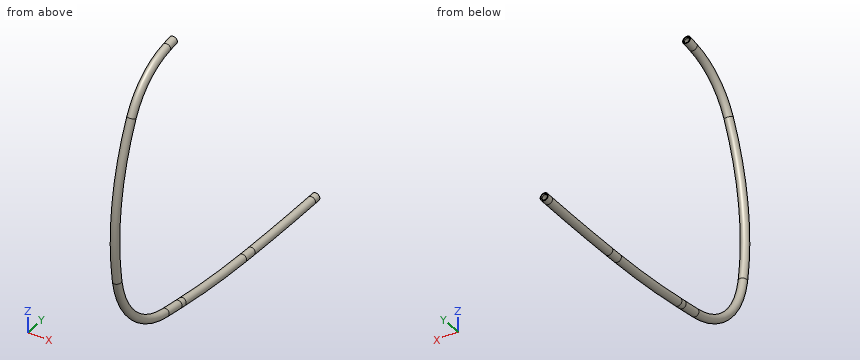
from build123d import *
from OCP.BRepFilletAPI import BRepFilletAPI_MakeChamfer

# Parameters (mm, degrees)
PERFIL_BOWDEN_R   = 3
PERFIL_BOWDEN_R_2 = 2
CHAFL_N2_SIZE     = 0.4
CHAFL_N2_SIZE2    = 0.692820323


with BuildPart() as part:
    # Barrer1: sweep along a curve in space
    with BuildLine() as barrer1_path:
        Line((-179.55, 237.9, 23.45), (-179.55, 232.9, 23.45))
        ThreePointArc((-179.55, 232.9, 23.45), (-179.55, 197.994333352, 23.830077258), (-179.55, 163.105218927, 24.970128802))
        ThreePointArc((-179.55, 163.105218927, 24.970128802), (-179.55, 158.110113707, 25.191344172), (-179.55, 153.115325109, 25.419596817))
        ThreePointArc((-179.55, 153.115325109, 25.419596817), (-179.55, 117.985550969, 28.025652191), (-179.55, 83.053766812, 32.571310699))
        Line((-179.55, 78.115325109, 33.353483024), (-179.55, 83.053766812, 32.571310699))
        Line((-179.55, 78.115325109, 33.353483024), (-179.55, 63.3, 35.7))
        ThreePointArc((-179.55, 63.3, 35.7), (-179.431411326, 26.758540491, 54.415674643), (-179.12153359, 8.351916444, 91.11266322))
        ThreePointArc((-179.12153359, 8.351916444, 91.11266322), (-178.587827908, 8.648566253, 149.248196445), (-178.054412898, 26.525914631, 204.567532573))
        ThreePointArc((-177.721385977, 68.000031071, 234.303977662), (-177.846418952, 43.604990817, 224.537163783), (-178.054412898, 26.525914631, 204.567532573))
        Line((-177.7, 75.8, 235.4), (-177.721385977, 68.000031071, 234.303977662))
    # Perfil bowden → Barrer1 (sweep)
    with BuildSketch(Plane(origin=(-179.55, 237.9, 23.45), x_dir=(-1, 0, 0), z_dir=(0, -1, 0))):
        Circle(PERFIL_BOWDEN_R)
        Circle(PERFIL_BOWDEN_R_2, mode=Mode.SUBTRACT)
    sweep(path=barrer1_path.line)

    # Chaflán2: one chamfer whose edges measure the first distance from different faces: ONE call of the kernel's chamfer builder (chamfer() names one face for all edges)
    chafl_n2_edges_1 = [part.edges().sort_by_distance(p)[0] for p in [
        (-175.700337449, 75.799679414, 235.363263359),
    ]]
    chafl_n2_side_1 = [part.faces().sort_by_distance(p)[0] for p in [
        (-174.785344671, 75.799532723, 235.346453642),
    ]]
    chafl_n2_edges_2 = [part.edges().sort_by_distance(p)[0] for p in [
        (-177.55, 237.9, 23.45),
    ]]
    chafl_n2_side_2 = [part.faces().sort_by_distance(p)[0] for p in [
        (-176.634852814, 237.9, 23.45),
    ]]
    chafl_n2 = BRepFilletAPI_MakeChamfer(part.part.solid().wrapped)
    for e in chafl_n2_edges_1:
        chafl_n2.Add(CHAFL_N2_SIZE, CHAFL_N2_SIZE2, e.wrapped, chafl_n2_side_1[0].wrapped)  # the first distance lies on this face
    for e in chafl_n2_edges_2:
        chafl_n2.Add(CHAFL_N2_SIZE, CHAFL_N2_SIZE2, e.wrapped, chafl_n2_side_2[0].wrapped)  # the first distance lies on this face
    add(Compound.cast(chafl_n2.Shape()), mode=Mode.REPLACE)


with BuildPart() as body_2:
    # Simetría2: mirrored copy
    add(part.part.mirror(Plane(origin=(0, 0, 0), x_dir=(0, 0, 1), z_dir=(1, 0, 0))))


solid = body_2.part
Model file for the job. Use its own axes, mm. Round coordinates to 2 decimals unless told otherwise and drop trailing zeros.
1. Drop flat-ended pins along their axis: P1, Ø1.5, axis at x = 176.5, z = 94, coming from the -Y side; P2, Ø1, axis at x = 181, z = 198, coming from the -Y side; P3, Ø3, axis at x = 180, y = 158, coming from the -Z side. Give the stop position or say it passes through.
Check values:
P1: stops at y = 5.54
P2: stops at y = 21.33
P3: stops at z = 22.13
2. Wall check: probe 1 along X at (y, z) = (233, 23); probe 2 along Z at (x, y) = (179.55, 234.3); probe 3 along Z at (x, y) = (179.25, 56). Give the ranges that are in metal, low to high.
Check values:
probe 1: x = 176.58 to 177.6, 181.5 to 182.52
probe 2: z = 20.45 to 21.45, 25.45 to 26.45
probe 3: z = 34.19 to 35.23, 39.34 to 40.39, 228.4 to 229.77, 232.64 to 233.99
3. Band-saw the part on A-A, the plane y = 58. Count the separate pieces of the cut face and the enclosed holes in it, and give its area (3 significant figures).
Check values:
separate pieces: 2
enclosed holes: 2
area: 32.8 mm2
